Work out the finished part from the listing and answer in its coordinate system (mm). A direction names the side the tool comes from. Give positions to 0.01 mm unless a question says otherwise; leave off trailing zeros. Order: outer loops, then holes, each group sorted by start corner. A loop starts at its lowest first (then second) coordinate and runs counter-clockwise, first axis right, second up. Notation, with made-up numbers: (74.25, -25.75) -> (85.25, -25.75) arc R16 ccw to (85.25, -6.75) -> close; hole circle Ø7 at (-12.5, 9). An arc over 180 degrees is marked (long way). Use a Markdown table: item, result. Add a question column.
Autodesk Inventor part; units mm, degrees
ref_plane "YZ Plane" through (0, 0, 0) normal (1, 0, 0) x (0, 1, 0)
ref_plane "XZ Plane" through (0, 0, 0) normal (0, 1, 0) x (-1, 0, 0)
ref_plane "XY Plane" through (0, 0, 0) normal (0, 0, 1) x (1, 0, 0)
sketch "Sketch1" plane through (0, 0, 0) normal (0, 0, 1) x (1, 0, 0)
  line L0 (0, 0) -> (44, 0)
  line L1 (44, 0) -> (44, 40)
  line L2 (44, 40) -> (0, 40)
  line L3 (0, 40) -> (0, 0)
  dimension "d0" = 44
  dimension "d1" = 40
extrude "Extrusion1" add sketch "Sketch1" along normal blind 82
sketch "Sketch2" plane through (0, 0, 0) normal (0, -1, 0) x (1, 0, 0)
  line L0 (6.8, 77.2) -> (37.2, 77.2)
  line L1 (37.2, 77.2) -> (37.2, 46.8)
  line L2 (37.2, 46.8) -> (6.8, 46.8)
  line L3 (6.8, 46.8) -> (6.8, 77.2)
  line L4 (0, 0) -> (0, 82)
  line L5 (0, 82) -> (44, 82)
  dimension "d4" = 30.4
  dimension "d5" = 30.4
  dimension "d6" = 6.8
  dimension "d7" = 4.8
extrude "Extrusion2" cut sketch "Sketch2" against normal blind 50
sketch "Sketch6" plane through (44, 0, 0) normal (1, 0, 0) x (0, 0, -1)
  circle A0 centre (-62.2, 30) radius 2.5
  circle A1 centre (-62.2, 10) radius 2.5
  line L0 (0, 40) -> (-82, 40)
  line L1 (0, 0) -> (-82, 0)
  point P0 (-77.2, 40)
  dimension "d24" = 5
  dimension "d25" = 10
  dimension "d26" = 5
  dimension "d27" = 10
  dimension "d28" = 15
  dimension "d29" = 15
extrude "Extrusion5" cut sketch "Sketch6" against normal blind 120
sketch "Sketch8" plane through (0, 0, 0) normal (-1, 0, 0) x (0, 0, 1)
  line L0 (0, 0) -> (0, 40)
  line L1 (77.2, 40) -> (46.8, 40)
  line L2 (0, 0) -> (82, 0)
  line L3 (82, 0) -> (82, 40)
  line L4 (82, 40) -> (0, 40)
  line L5 (0, 40) -> (0, 0)
  line L6 (82, 40) -> (82, 0)
extrude "Extrusion7" add sketch "Sketch8" along normal blind 45
sketch "Sketch4" plane through (44, 0, 0) normal (1, 0, 0) x (0, 0, -1)
  line L0 (-6, 7.1) -> (-46.8, 7.1)
  line L1 (-46.8, 7.1) -> (-46.8, 32.9)
  line L2 (-46.8, 32.9) -> (-6, 32.9)
  line L3 (-6, 32.9) -> (-6, 7.1)
  line L4 (0, 0) -> (0, 40)
  line L5 (0, 0) -> (-82, 0)
  line L6 (-46.8, 0) -> (-46.8, 40)
  point P0 (0, 20)
  point P1 (-6, 20)
  dimension "d10" = 25.8
  dimension "d11" = 40.8
  dimension "d13" = 7.1
extrude "Extrusion3" cut sketch "Sketch4" against normal blind 84
sketch "Sketch5" plane through (0, 0, 0) normal (0, 0, -1) x (-1, 0, 0)
  circle A0 centre (34.2, 20) radius 3.1
  circle A1 centre (15.2, 20) radius 3.1
  line L0 (-44, 40) -> (0, 40)
  line L1 (45, 40) -> (45, 0)
  point P0 (0, 0)
  dimension "d16" = 6.2
  dimension "d17" = 6.2
  dimension "d18" = 20
  dimension "d19" = 20
  dimension "d21" = 19
  dimension "d40" = 10.8
extrude "Extrusion4" cut sketch "Sketch5" against normal blind 34
sketch "Sketch9" plane through (44, 7.1, 6) normal (0, 0, 1) x (1, 0, 0)
  line L0 (0, 25.8) -> (-84, 25.8)
  line L1 (0, 0) -> (-84, 0)
  line L2 (0, 25.8) -> (-50, 25.8)
  line L3 (-50, 25.8) -> (-50, 0)
  line L4 (-50, 0) -> (0, 0)
  line L5 (0, 0) -> (0, 25.8)
  line L6 (-84, 25.8) -> (-84, 0)
  point P0 (-44, -7.1)
  point P1 (-50, 25.8)
  point P2 (-84, 0)
  dimension "d41" = 34
extrude "Extrusion8" cut sketch "Sketch9" against normal blind 10 contours L5 L1 L3 L0
sketch "Sketch10" plane through (44, 0, 82) normal (1, 0, 0) x (0, 0, -1)
  line L0 (33.2, 5.1) -> (82, 5.1)
  line L1 (82, 5.1) -> (82, 34.9)
  line L2 (82, 34.9) -> (33.2, 34.9)
  line L3 (33.2, 34.9) -> (33.2, 5.1)
  line L4 (35.2, 7.1) -> (35.2, 32.9)
  line L5 (82, 7.1) -> (35.2, 7.1)
  line L6 (35.2, 32.9) -> (82, 32.9)
  point P0 (82, 0)
  dimension "d44" = 2
  dimension "d45" = 2
  dimension "d46" = 2
extrude "Extrusion9" cut sketch "Sketch10" against normal up to surface (50 mm away) contours L3 L2 L1 L6 L4 L5 L0
fillet "Fillet1" radius 40 3 edges at (44, 2.55, 0) (44, 37.45, 0) (-45, 20, 82)
sketch "Sketch11" plane through (-40, 0, 0) normal (1, 0, 0) x (0, 0, -1)
  circle A0 centre (-31, 20.4) radius 3.5
  line L0 (-6, 32.9) -> (0, 32.9)
  line L1 (-6, 7.1) -> (-6, 32.9)
  line L2 (-46.8, 32.9) -> (-6, 32.9)
  point P0 (0, 0)
  point P1 (-46.8, 32.7)
  point P2 (-6, 20)
  point P3 (0, 32.9)
  dimension "d50" = 7
  dimension "d52" = 25
  dimension "d55" = 12.5
extrude "Extrusion10" cut sketch "Sketch11" against normal blind 109
sketch "Sketch12" plane through (0, 30, 62.2) normal (1, 0, 0) x (0, 0, -1)
  circle A0 centre (0, 0) radius 6
  circle A1 centre (0, -20) radius 6
  circle A2 centre (0, -20) radius 2.5
  circle A3 centre (0, 0) radius 2.5
  point P0 (62.2, -30)
  dimension "d56" = 12
  dimension "d57" = 12
extrude "Extrusion11" cut sketch "Sketch12" against normal blind 120 contours A0 | A1 | A2 | A3
properties part number "loacell_mount2"
1) The part is cut by section D-D, the plane z = 44. Determine the outline of the cut face in (x, y), then the cut area to 3 significant figures.
2) The part is cut by section C-C, the plane z = 62.2. State how many separate pieces and enclosed holes the cut face has, then the cut area to 3 significant figures.
3) Determine the mould class of faces 1 (the flat face through (-40, 20, 27)), 2 (the flat face through (6.8, 20, 62)), 3 (the cylindrical face through (32.594, 2.586, 12.028)), 4 (the flat face through (-6, 33.3, 19.1)) for opening direction Z: released by +Z, released by -Z, zero draft, split by the parting line, or undercut.
4) Flat-ended cylindrical pins translate along their axes: pin 1 (7.5 mm diameter, centred on x = 41.5, y = 26.5, fed in from -Z); pin 2 (1 mm diameter, centred on y = 15.5, z = 39, fed in from +X); pin 3 (5.5 mm diameter, centred on x = -34.2, y = 20, fed in from -Z); pin 4 (3 mm diameter, centred on y = 10, z = 62.2, fed in from -X). Find the tip coordinate at first contact, or state that the pin passes through.
5) Straight lines are drawn through the part: line 1 (Y direction, x = -26, z = 62.2); line 2 (Y direction, x = 3, z = 62); line 3 (Z direction, x = -9, y = 10). For each, find the intervals that lie inside material, in ascending order.
6) Which of the six approach directions +Z, -Z, +X, -X, +Y, -Y give full straight-line access (tool end or side, diameter ignored) to faces 5 (the flat face through (22, 37, 46.8)), 6 (the cylindrical face through (-12.74, 18.114, 2.958)), 7 (the flat face through (0, 20, 48.8)), 8 (the flat face through (0, 27, 62))?
7) The part is cut by section B-B, the plane y = 30. Determine the outline of the cut face in (x, z).
8) The part is cut by section A-A, the plane x = 10.5. Determine the outline of the cut face in (y, z), then the cut area to 3 significant figures.
A:
| question | item | result |
|---|---|---|
| 1 | outline | (-44.95, 0) -> (44, 0) -> (44, 5.1) -> (-6, 5.1) -> (-6, 7.1) -> (-40, 7.1) -> (-40, 32.9) -> (-6, 32.9) -> (-6, 34.9) -> (44, 34.9) -> (44, 40) -> (-44.95, 40) -> close |
| 1 | area | 1,190 mm^2 |
| 2 | separate pieces | 6 |
| 2 | enclosed holes | 0 |
| 2 | area | 1,040 mm^2 |
| 3 | face 1 | undercut |
| 3 | face 2 | undercut |
| 3 | face 3 | released by -Z |
| 3 | face 4 | zero draft |
| 4 | pin 1 | z = 48.8 |
| 4 | pin 2 | x = -40 |
| 4 | pin 3 | z = 46.8 |
| 4 | pin 4 | through |
| 5 | line 1 | 0 to 4, 16 to 24, 36 to 40 |
| 5 | line 2 | 0 to 7.51, 12.49 to 27.51, 32.49 to 40 |
| 5 | line 3 | 0 to 6, 46.8 to 56.2, 68.2 to 81.8 |
| 6 | face 5 | +Y, -Y |
| 6 | face 6 | -Z |
| 6 | face 7 | -Z, +X |
| 6 | face 8 | -X |
| 7 | outline | (-45, 0) -> (-6, 0) -> (-6, 6) -> (-40, 6) -> (-40, 46.8) -> (-6, 46.8) -> (-6, 48.8) -> (6.8, 48.8) -> (6.8, 59.7) -> (0, 59.7) -> (0, 56.2) -> (-42.39, 56.2) arc R40 ccw to (-45, 42) -> close; (-35.23, 68.2) -> (0, 68.2) -> (0, 64.7) -> (6.8, 64.7) -> (6.8, 77.2) -> (37.2, 77.2) -> (37.2, 64.7) -> (44, 64.7) -> (44, 82) -> (-5, 82) arc R40 ccw to start; (37.2, 48.8) -> (44, 48.8) -> (44, 59.7) -> (37.2, 59.7) -> close |
| 8 | outline | (0, 0.53) -> (5.1, 0.53) -> (5.1, 46.8) -> (0, 46.8) -> close; (0, 77.2) -> (40, 77.2) -> (40, 82) -> (0, 82) -> close; (34.9, 0.53) -> (40, 0.53) -> (40, 46.8) -> (34.9, 46.8) -> close |
| 8 | area | 664 mm^2 |
